Input: part model. Units: mm. Frame: model coordinates. Face numbers are marked on the shaded views. A direction names the side the tool comes from. Coordinates: 2 decimals unless noted, no trailing zeros. Write each loop counter-clockwise with the first axis right and the second up, starting at its lowest first coordinate (ties: lowest second). Pieces come first, ordered by that corner, then holes. Notation, with made-up numbers: (-10, 51.25) - (18, 51.25) arc R22 cw to (18, 57.25) - close; hole circle Ø1 at (62.5, 60). An arc over 180 degrees is marked (long way). Put each result on its own line as item: value. Start each with the question number.
1. Access query for the marked faces 1, 2 and 3. Directions: +Z, -Z, +X, -X, +Y, -Y. A direction counts if a zero-diameter tool reaches every point of the face in a straight line with its end or side. Return the directions, or none.
2. Line query: line 1 (Y direction, x = 2.5, z = -4.5) (3 decimals); line 2 (Y direction, x = -3.5, z = 3.75) (3 decimals); line 3 (X direction, y = 0.25, z = -1.75) (3 decimals). Output: solid intervals per line, ascending.
3. Pin query (flat end, axial travel): pin 1 (4 mm diameter, centred on x = 0.5, z = -0.5, fed in from -Y) (3 decimals); pin 2 (0.8 mm diameter, centred on y = -4.5, z = -2.5, fed in from +X); pin 3 (1.1 mm diameter, centred on x = 3.5, z = 3.5, fed in from +Y) (3 decimals). Return the tip coordinate at first contact, or that it passes through.
4. Cut plane D-D, the plane y = 3.5. Return loops of the section in (x, z) (3 decimals), and give its area (3 significant figures).
5. Cut plane A-A, the plane y = -2.25. Return loops of the section in (x, z), and give its area (3 significant figures).
from build123d import *

# Parameters (mm, degrees)
SKETCH1_W               = 11.93
SKETCH1_H               = 11.93
BOSS_EXTRUDE1_DEPTH     = 1.575
CUT_EXTRUDE_THIN1_DEPTH = 0.1
SKETCH3_R               = 0.75
BOSS_EXTRUDE2_DEPTH     = 0.1
FILLET1_R               = 0.05
SKETCH4_R               = 3.335
BOSS_EXTRUDE3_DEPTH     = 2.7
EXTRUDE_THIN1_DEPTH     = 11.92
SKETCH6_W               = 4
SKETCH6_H               = 7.725942516
SKETCH6_W_2             = 4.750048421
CUT_EXTRUDE1_DEPTH      = 16.26080664
SKETCH7_W               = 4.750048421
SKETCH7_H               = 7.725942516
SKETCH7_W_2             = 4
CUT_EXTRUDE2_DEPTH      = 16.26080664


with BuildPart() as part:
    # Sketch1 → Boss-Extrude1 (new, symmetric)
    with BuildSketch(Plane(origin=(0, 0, 0), x_dir=(1, 0, 0), z_dir=(0, 1, 0))):
        Rectangle(SKETCH1_W, SKETCH1_H)
    extrude(amount=BOSS_EXTRUDE1_DEPTH, both=True)

    # Sketch2 → Cut-Extrude-Thin1 (cut)
    with BuildSketch(Plane(origin=(0, 1.575, 0), x_dir=(1, 0, 0), z_dir=(0, 1, 0))):
        with BuildLine():
            Line((4.465, 4.7775), (-4.465, 4.7775))
            ThreePointArc((-4.465, 4.7775), (-4.685970869, 4.685970869), (-4.7775, 4.465))
            Line((-4.7775, 4.465), (-4.7775, -4.465))
            ThreePointArc((-4.7775, -4.465), (-4.685970869, -4.685970869), (-4.465, -4.7775))
            Line((-4.465, -4.7775), (4.465, -4.7775))
            ThreePointArc((4.465, -4.7775), (4.685970869, -4.685970869), (4.7775, -4.465))
            Line((4.7775, -4.465), (4.7775, 4.465))
            ThreePointArc((4.7775, 4.465), (4.685970869, 4.685970869), (4.465, 4.7775))
        make_face()
        with BuildLine():
            Line((4.465, 4.6525), (-4.465, 4.6525))
            ThreePointArc((-4.465, 4.6525), (-4.597582521, 4.597582521), (-4.6525, 4.465))
            Line((-4.6525, 4.465), (-4.6525, -4.465))
            ThreePointArc((-4.6525, -4.465), (-4.597582521, -4.597582521), (-4.465, -4.6525))
            Line((-4.465, -4.6525), (4.465, -4.6525))
            ThreePointArc((4.465, -4.6525), (4.597582521, -4.597582521), (4.6525, -4.465))
            Line((4.6525, -4.465), (4.6525, 4.465))
            ThreePointArc((4.6525, 4.465), (4.597582521, 4.597582521), (4.465, 4.6525))
        make_face(mode=Mode.SUBTRACT)
    extrude(amount=-CUT_EXTRUDE_THIN1_DEPTH, mode=Mode.SUBTRACT)

    # Sketch3 → Boss-Extrude2 (add)
    with BuildSketch(Plane(origin=(0, 1.575, 0), x_dir=(1, 0, 0), z_dir=(0, 1, 0))):
        with Locations(Location((-3.625, 3.625, 0), (0, 0, 270))):
            Circle(SKETCH3_R)
        with Locations(Location((3.625, 3.625, 0), (0, 0, 270))):
            Circle(SKETCH3_R)
        with Locations(Location((3.625, -3.625, 0), (0, 0, 270))):
            Circle(SKETCH3_R)
        with Locations(Location((-3.625, -3.625, 0), (0, 0, 270))):
            Circle(SKETCH3_R)
    extrude(amount=BOSS_EXTRUDE2_DEPTH)

    # Fillet1
    fillet1_edges = [part.edges().sort_by_distance(p)[0] for p in [
        (-3.625, 1.675, -4.375),
        (3.625, 1.675, -4.375),
        (3.625, 1.675, 2.875),
        (-3.625, 1.675, 2.875),
    ]]
    fillet(fillet1_edges, radius=FILLET1_R)

    # Sketch4 → Boss-Extrude3 (add)
    with BuildSketch(Plane(origin=(0, 1.575, 0), x_dir=(1, 0, 0), z_dir=(0, 1, 0))):
        with Locations(Location((0, 0, 0), (0, 0, 90))):
            Circle(SKETCH4_R)
    extrude(amount=BOSS_EXTRUDE3_DEPTH)

    # Sketch5 → Extrude-Thin1 (add)
    with BuildSketch(Plane.XY.offset(5.965)):
        Polygon((-6.3025, -5.075), (-6.3025, -4.303555766), (-6.997085308, -3.410517513), (-6.315993287, -0.6375), (6.315993287, -0.6375), (6.997085308, -3.410517513), (6.3025, -4.303555766), (6.3025, -5.075), (6.4275, -5.075), (6.4275, -4.346444234), (7.132914692, -3.439482487), (6.414006713, -0.5125), (-6.414006713, -0.5125), (-7.132914692, -3.439482487), (-6.4275, -4.346444234), (-6.4275, -5.075), align=None)
    extrude(amount=-EXTRUDE_THIN1_DEPTH)

    # Sketch6 → Cut-Extrude1 (cut, through all)
    with BuildSketch(Plane(origin=(5.965, 0, 0), x_dir=(0, 0, -1), z_dir=(1, 0, 0))):
        with Locations((0, -1.737877721)):
            Rectangle(SKETCH6_W, SKETCH6_H)
        with Locations((-5.375024211, -1.737877721)):
            Rectangle(SKETCH6_W_2, SKETCH6_H)
        with Locations((5.375024211, -1.737877721)):
            Rectangle(SKETCH6_W_2, SKETCH6_H)
    extrude(amount=CUT_EXTRUDE1_DEPTH, mode=Mode.SUBTRACT)

    # Sketch7 → Cut-Extrude2 (cut, through all)
    with BuildSketch(Plane.ZY.offset(5.965)):
        with Locations((-5.375024211, -1.737877721)):
            Rectangle(SKETCH7_W, SKETCH7_H)
        with Locations((5.375024211, -1.737877721)):
            Rectangle(SKETCH7_W, SKETCH7_H)
        with Locations((0, -1.737877721)):
            Rectangle(SKETCH7_W_2, SKETCH7_H)
    extrude(amount=CUT_EXTRUDE2_DEPTH, mode=Mode.SUBTRACT)


solid = part.part
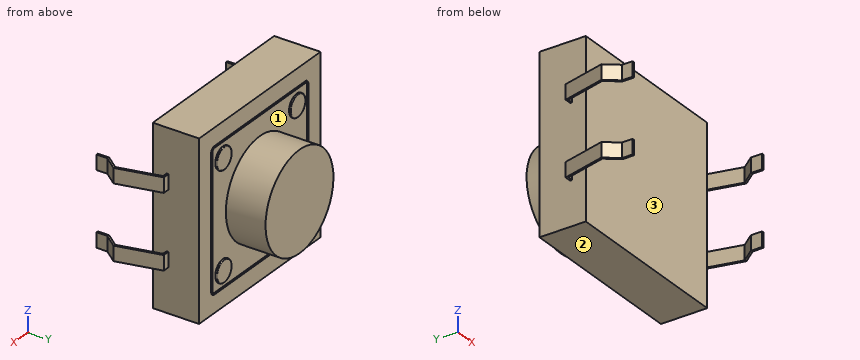
Report:
1. face 1: +Y
1. face 2: -Z, +X, -X, +Y, -Y
1. face 3: +Z, -Z, -Y
2. line 1: y = -1.575 to 1.575
2. line 2: y = -1.575 to 1.675
2. line 3: x = -5.965 to 5.965
3. pin 1: stops at y = -1.575
3. pin 2: stops at x = 6.62
3. pin 3: stops at y = 1.675
4. outline: circle Ø6.67 at (0, 0)
4. area: 34.9 mm^2
5. outline: (-6.84, -3) - (-6.71, -3) - (-6.71, -2) - (-6.84, -2) - close; (-6.84, 2) - (-6.71, 2) - (-6.71, 3) - (-6.84, 3) - close; (6.71, -3) - (6.84, -3) - (6.84, -2) - (6.71, -2) - close; (6.71, 2) - (6.84, 2) - (6.84, 3) - (6.71, 3) - close
5. area: 0.515 mm^2
